The model under review builds one solid part; all positions refer to its coordinate system, in mm. Face numbers are marked on the shaded views. A direction names the side the tool comes from. Round coordinates to 2 decimals unless told otherwise and drop trailing zeros. Order: outer loops, then holes, each group sorted by start corner. A loop starts at its lowest first (then second) coordinate and runs counter-clockwise, first axis right, second up. Notation, with made-up numbers: M -26,-20.5 L -13,-20.5 A14 ccw -13,-4.5 Z; hole C -15,21.25 d3. An arc over 180 degrees is marked long. Answer as a JSON object with one key per item and string values. Group by question number.
1) Consider section A-A, the plane x = 0. Write out the cut boundary in (y, z) (3 decimals), then the cut area to 3 significant figures.
2) To check wall thickness, follow line 1 (Z direction, x = 0, y = 1.45) (3 decimals); line 2 (Z direction, x = -25, y = 8.75) (3 decimals); line 3 (Y direction, x = 6, z = -21). State the ranges of each line that lie inside material, in increasing order.
3) Consider section B-B, the plane y = 13.75. Write out the cut boundary in (x, z) (3 decimals), then the cut area to 3 significant figures.
4) Consider section D-D, the plane x = -8.8. Write out the cut boundary in (y, z) (3 decimals).
5) For the marked faces 1, 2 and 3, list the 3-axis set-ups (+Z, -Z, +X, -X, +Y, -Y) from which the entire face can be reached by the end or side of a thin tool; tool diameter is ignored.
6) Insertion check: pin 1 Ø3 at (y, z) = (10.5, -22.5) entering from -X; pin 2 Ø5.5 at (x, y) = (-23, 11.5) entering from -Z (3 decimals); pin 3 Ø1.5 at (x, z) = (-8.8, 20.18) entering from -Y; pin 4 Ø12 at (x, z) = (3.5, 10.5) entering from +Y. Each pin has a flat end and moves straight along its axis. Give the tip position at first contact, or say it passes through.
7) Consider section C-C, the plane x = 22.86. Write out the cut boundary in (y, z) (3 decimals), then the cut area to 3 significant figures.
8) The part is to be moulded in two halves that separate along X. For the marked faces 4, 5, 6 and 7, say which applies: +X half, -X half, draft (parallel to the pull), parting line (faces both ways), or undercut.
```python
from build123d import *

# Parameters (mm, degrees)
SKETCH2_W           = 54.8
SKETCH2_H           = 53.53
BOSS_EXTRUDE1_DEPTH = 2
SKETCH3_W           = 5.08
SKETCH3_H           = 6.35
BOSS_EXTRUDE2_DEPTH = 13
SKETCH6_R           = 1.25
BOSS_EXTRUDE3_DEPTH = 5
CUT_EXTRUDE1_REACH  = 22
SKETCH7_W           = 13.1
SKETCH7_H           = 7.1
CUT_EXTRUDE2_REACH  = 22
SKETCH8_R           = 1.25
CUT_EXTRUDE4_REACH  = 54.8
SKETCH9_R           = 0.625
CUT_EXTRUDE5_REACH  = 54.8
SKETCH10_R          = 0.625
CUT_EXTRUDE6_REACH  = 54.8
SKETCH11_R          = 0.625
CUT_EXTRUDE7_REACH  = 4
SKETCH12_R          = 1.25
CUT_EXTRUDE8_REACH  = 4
SKETCH13_R          = 1.25


with BuildPart() as part:
    # Sketch2 → Boss-Extrude1 (new body)
    with BuildSketch(Plane(origin=(0, 0, 0), x_dir=(1, 0, 0), z_dir=(0, 1, 0))):
        Rectangle(SKETCH2_W, SKETCH2_H)
    extrude(amount=BOSS_EXTRUDE1_DEPTH)

    # Sketch3 → Boss-Extrude2 (add)
    with BuildSketch(Plane(origin=(0, 2, 0), x_dir=(1, 0, 0), z_dir=(0, 1, 0))):
        with Locations((-22.86, 21.59)):
            Rectangle(SKETCH3_W, SKETCH3_H)
        with Locations((22.86, 21.59)):
            Rectangle(SKETCH3_W, SKETCH3_H)
        with Locations((-22.86, -21.59)):
            Rectangle(SKETCH3_W, SKETCH3_H)
    extrude(amount=BOSS_EXTRUDE2_DEPTH)

    # Sketch6 → Boss-Extrude3 (add)
    with BuildSketch(Plane(origin=(0, 15, 0), x_dir=(1, 0, 0), z_dir=(0, 1, 0))):
        with Locations((-22.86, 22.225)):
            Circle(SKETCH6_R)
        with Locations((22.86, 22.225)):
            Circle(SKETCH6_R)
        with Locations((-22.86, -22.225)):
            Circle(SKETCH6_R)
    extrude(amount=BOSS_EXTRUDE3_DEPTH)

    # Sketch7 → Cut-Extrude1 (cut, up to next)
    with BuildSketch(Plane(origin=(0, 0, 0), x_dir=(-1, 0, 0), z_dir=(0, -1, 0)), mode=Mode.PRIVATE) as cut_extrude1_sk1:
        with Locations((0, -20.180596319)):
            Rectangle(SKETCH7_W, SKETCH7_H)
    cut_extrude1_tool1 = extrude(cut_extrude1_sk1.sketch, amount=-CUT_EXTRUDE1_REACH, mode=Mode.PRIVATE) & part.part
    add(cut_extrude1_tool1.solids().sort_by_distance((0, 0, 20.180596))[0], mode=Mode.SUBTRACT)

    # Sketch8 → Cut-Extrude2 (cut, up to next)
    with BuildSketch(Plane.XZ, mode=Mode.PRIVATE) as cut_extrude2_sk1:
        with Locations((0, 6.530805807)):
            Circle(SKETCH8_R)
    cut_extrude2_tool1 = extrude(cut_extrude2_sk1.sketch, amount=-CUT_EXTRUDE2_REACH, mode=Mode.PRIVATE) & part.part
    add(cut_extrude2_tool1.solids().sort_by_distance((0, 0, 6.530806))[0], mode=Mode.SUBTRACT)
    # Sketch8 → Cut-Extrude2 (cut, up to next)
    with BuildSketch(Plane.XZ, mode=Mode.PRIVATE) as cut_extrude2_sk2:
        with Locations((0, -16.969194193)):
            Circle(SKETCH8_R)
    cut_extrude2_tool2 = extrude(cut_extrude2_sk2.sketch, amount=-CUT_EXTRUDE2_REACH, mode=Mode.PRIVATE) & part.part
    add(cut_extrude2_tool2.solids().sort_by_distance((0, 0, -16.969194))[0], mode=Mode.SUBTRACT)

    # Sketch9 → Cut-Extrude4 (cut, up to next)
    with BuildSketch(Plane.ZY.offset(25.4), mode=Mode.PRIVATE) as cut_extrude4_sk1:
        with Locations((-21.59, 7.11470595)):
            Circle(SKETCH9_R)
    cut_extrude4_tool1 = extrude(cut_extrude4_sk1.sketch, amount=-CUT_EXTRUDE4_REACH, mode=Mode.PRIVATE) & part.part
    add(cut_extrude4_tool1.solids().sort_by_distance((-25.4, 7.114706, -21.59))[0], mode=Mode.SUBTRACT)

    # Sketch10 → Cut-Extrude5 (cut, up to next)
    with BuildSketch(Plane(origin=(25.4, 0, 0), x_dir=(0, 0, -1), z_dir=(1, 0, 0)), mode=Mode.PRIVATE) as cut_extrude5_sk1:
        with Locations((21.595, 7.11)):
            Circle(SKETCH10_R)
    cut_extrude5_tool1 = extrude(cut_extrude5_sk1.sketch, amount=-CUT_EXTRUDE5_REACH, mode=Mode.PRIVATE) & part.part
    add(cut_extrude5_tool1.solids().sort_by_distance((25.4, 7.11, -21.595))[0], mode=Mode.SUBTRACT)

    # Sketch11 → Cut-Extrude6 (cut, up to next)
    with BuildSketch(Plane.ZY.offset(25.4), mode=Mode.PRIVATE) as cut_extrude6_sk1:
        with Locations((21.595, 7.11)):
            Circle(SKETCH11_R)
    cut_extrude6_tool1 = extrude(cut_extrude6_sk1.sketch, amount=-CUT_EXTRUDE6_REACH, mode=Mode.PRIVATE) & part.part
    add(cut_extrude6_tool1.solids().sort_by_distance((-25.4, 7.11, 21.595))[0], mode=Mode.SUBTRACT)

    # Sketch12 → Cut-Extrude7 (cut, up to next)
    with BuildSketch(Plane(origin=(0, 2, 0), x_dir=(1, 0, 0), z_dir=(0, 1, 0)), mode=Mode.PRIVATE) as cut_extrude7_sk1:
        with Locations((-14.835465402, -17.017151491)):
            Circle(SKETCH12_R)
    cut_extrude7_tool1 = extrude(cut_extrude7_sk1.sketch, amount=-CUT_EXTRUDE7_REACH, mode=Mode.PRIVATE) & part.part
    add(cut_extrude7_tool1.solids().sort_by_distance((-14.835465, 2, 17.017151))[0], mode=Mode.SUBTRACT)

    # Sketch13 → Cut-Extrude8 (cut, up to next)
    with BuildSketch(Plane(origin=(0, 2, 0), x_dir=(1, 0, 0), z_dir=(0, 1, 0)), mode=Mode.PRIVATE) as cut_extrude8_sk1:
        with Locations((-8.8, -20.180596319)):
            Circle(SKETCH13_R)
    cut_extrude8_tool1 = extrude(cut_extrude8_sk1.sketch, amount=-CUT_EXTRUDE8_REACH, mode=Mode.PRIVATE) & part.part
    add(cut_extrude8_tool1.solids().sort_by_distance((-8.8, 2, 20.180596))[0], mode=Mode.SUBTRACT)
    # Sketch13 → Cut-Extrude8 (cut, up to next)
    with BuildSketch(Plane(origin=(0, 2, 0), x_dir=(1, 0, 0), z_dir=(0, 1, 0)), mode=Mode.PRIVATE) as cut_extrude8_sk2:
        with Locations((8.7, -20.180596319)):
            Circle(SKETCH13_R)
    cut_extrude8_tool2 = extrude(cut_extrude8_sk2.sketch, amount=-CUT_EXTRUDE8_REACH, mode=Mode.PRIVATE) & part.part
    add(cut_extrude8_tool2.solids().sort_by_distance((8.7, 2, 20.180596))[0], mode=Mode.SUBTRACT)


solid = part.part
```
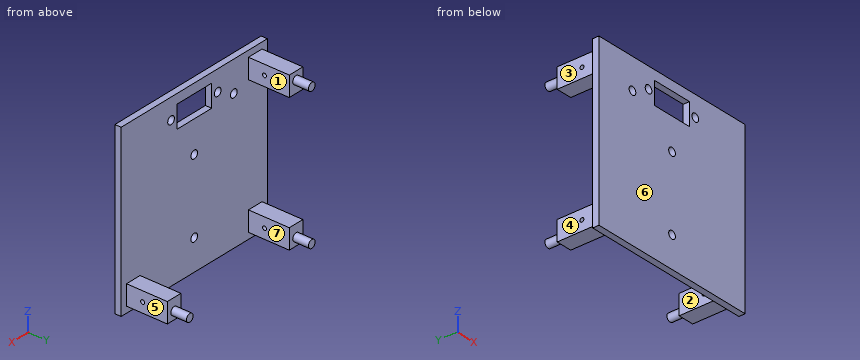
Results list:
{
 "1": {"outline": "M 0,-26.765 L 2,-26.765 L 2,-18.219 L 0,-18.219 Z; M 0,-15.719 L 2,-15.719 L 2,5.281 L 0,5.281 Z; M 0,7.781 L 2,7.781 L 2,16.631 L 0,16.631 Z; M 0,23.731 L 2,23.731 L 2,26.765 L 0,26.765 Z", "area": "82.9 mm^2"},
 "2": {"line 1": "-26.765 to -18.219, -15.719 to 5.281, 7.781 to 16.631, 23.731 to 26.765", "line 2": "-24.765 to -18.415, 18.415 to 24.765", "line 3": "0 to 2"},
 "3": {"outline": "M -25.4,-24.765 L -20.32,-24.765 L -20.32,-18.415 L -25.4,-18.415 Z; M -25.4,18.415 L -20.32,18.415 L -20.32,24.765 L -25.4,24.765 Z; M 20.32,-24.765 L 25.4,-24.765 L 25.4,-18.415 L 20.32,-18.415 Z", "area": "96.8 mm^2"},
 "4": {"outline": "M 0,-26.765 L 2,-26.765 L 2,18.931 L 0,18.931 Z; M 0,21.431 L 2,21.431 L 2,26.765 L 0,26.765 Z"},
 "5": {"face 1": "+Z, -Z, +X, +Y", "face 2": "+Z, -Z, +Y", "face 3": "+Z, -Z, -X, +Y"},
 "6": {"pin 1": "x = -25.4", "pin 2": "z = -24.765", "pin 3": "through", "pin 4": "y = 2"},
 "7": {"outline": "M 0,-26.765 L 2,-26.765 L 2,-24.765 L 15,-24.765 L 15,-23.475 L 20,-23.475 L 20,-20.975 L 15,-20.975 L 15,-18.415 L 2,-18.415 L 2,26.765 L 0,26.765 Z; hole C 7.11,-21.595 d1.25", "area": "201 mm^2"},
 "8": {"face 4": "-X half", "face 5": "+X half", "face 6": "draft", "face 7": "undercut"}
}
